from build123d import *

# Parameters (mm, degrees)
BOSS_EXTRU_1_DEPTH      = 6
ESQUISSE2_R             = 17.5
ESQUISSE2_R_2           = 1.65
ENL_V_MAT_EXTRU_1_DEPTH = 107.283818147
ENL_V_MAT_EXTRU_3_DEPTH = 107.283818147
ESQUISSE6_R             = 3.5
ENL_V_MAT_EXTRU_4_DEPTH = 4
CONG_1_R                = 20


with BuildPart() as part:
    # Esquisse1 → Boss.-Extru.1 (new body)
    with BuildSketch(Plane(origin=(0, 0, 0), x_dir=(1, 0, 0), z_dir=(0, 1, 0))):
        Polygon((-94, -35.5), (-94, -25.5), (-100, -25.5), (-100, -10.5), (-94, -10.5), (-94, 10.5), (-100, 10.5), (-100, 25.5), (-94, 25.5), (-94, 35.5), (94, 35.5), (94, 25.5), (100, 25.5), (100, 10.5), (94, 10.5), (94, -10.5), (100, -10.5), (100, -25.5), (94, -25.5), (94, -35.5), align=None)
    extrude(amount=BOSS_EXTRU_1_DEPTH)

    # Esquisse2 → Enlèv. mat.-Extru.1 (cut, through all)
    with BuildSketch(Plane(origin=(0, 0, 0), x_dir=(-1, 0, 0), z_dir=(0, -1, 0))):
        with Locations(Location((18, 11.5, 0), (0, 0, 90))):
            Circle(ESQUISSE2_R)
        with Locations(Location((71, -24.5, 0), (0, 0, 90))):
            Circle(ESQUISSE2_R_2)
        with Locations(Location((71, 25.5, 0), (0, 0, 90))):
            Circle(ESQUISSE2_R_2)
        with Locations(Location((-71, 25.5, 0), (0, 0, 270))):
            Circle(ESQUISSE2_R_2)
        with Locations(Location((-71, -24.5, 0), (0, 0, 270))):
            Circle(ESQUISSE2_R_2)
        with Locations(Location((-18, 11.5, 0), (0, 0, 270))):
            Circle(ESQUISSE2_R)
    extrude(amount=-ENL_V_MAT_EXTRU_1_DEPTH, mode=Mode.SUBTRACT)

    # Esquisse5 → Enlèv. mat.-Extru.3 (cut, through all)
    with BuildSketch(Plane.XZ):
        Polygon((-31.565369037, -0.444197772), (-18, -29), (18, -29), (31.565369037, -0.444197772), (18.743702877, 19.662334717), (-17.256297123, 19.662334717), align=None)
    extrude(amount=-ENL_V_MAT_EXTRU_3_DEPTH, mode=Mode.SUBTRACT)

    # Esquisse6 → Enlèv. mat.-Extru.4 (cut)
    with BuildSketch(Plane(origin=(0, 6, 0), x_dir=(1, 0, 0), z_dir=(0, 1, 0))):
        with Locations(Location((71, -24.5, 0), (0, 0, 270))):
            Circle(ESQUISSE6_R)
        with Locations(Location((71, 25.5, 0), (0, 0, 270))):
            Circle(ESQUISSE6_R)
        with Locations(Location((-71, 25.5, 0), (0, 0, 270))):
            Circle(ESQUISSE6_R)
        with Locations(Location((-71, -24.5, 0), (0, 0, 270))):
            Circle(ESQUISSE6_R)
    extrude(amount=-ENL_V_MAT_EXTRU_4_DEPTH, mode=Mode.SUBTRACT)

    # Congé1
    cong_1_edges = [part.edges().sort_by_distance(p)[0] for p in [
        (-17.256297123, 3, 19.662334717),
        (18.743702877, 3, 19.662334717),
    ]]
    fillet(cong_1_edges, radius=CONG_1_R)


solid = part.part
For this review, take the finished solid that the model builds, in its own axes (mm). A direction names the side the tool comes from. Round coordinates to 2 decimals unless told otherwise and drop trailing zeros. Write each loop counter-clockwise with the first axis right and the second up, starting at its lowest first coordinate (ties: lowest second). Pieces come first, ordered by that corner, then holes. Notation, with made-up numbers: M 1,-14 L 20,-14 A32 cw 20,16 Z; hole C 89.25,37.5 d5. An arc over 180 degrees is marked long. Write item = value, one per line. Start each with the question number.
(1) Clearance check with flat-ended pins moving along their axes: pin 1 Ø3 at (x, y) = (-96, 3.5) entering from -Z; pin 2 Ø2 at (x, z) = (69.5, 23.5) entering from +Y; pin 3 Ø3 at (x, z) = (-71, -25.5) entering from +Y; pin 4 Ø3 at (y, z) = (2.5, -28.5) entering from +X. State where each tip first meets the part, or that it passes through.
(2) The part is to be moulded in two halves that separate along X. For faces 6 (the face through (100, 3, 18)), 7 (the face through (97, 3, 25.5)), 8 (the face through (-33.924, 2.958, -18.759)), say which applies: +X half, -X half, draft (parallel to the pull), parting line (faces both ways), or undercut.
(3) For line 1 along Z through (x, y) = (71, 0.7); line 2 along X through (y, z) = (0.8, 24.5); line 3 along X through (y, z) = (4, 22), list the stretches that pass through material, from the lowest coordinate up.
(4) We need section C-C (z = -17). Give the boundary of the cut face in (x, y).
(5) We need section A-A (x = 4). Give the boundary of the cut face in (y, z), then the cut area to 3 significant figures.
(6) For faces 1 (the face through (33.687, 2.958, -19.258)), 2 (the face through (-94, 3, -30)), 3 (the face through (97, 3, -10.5)), 4 (the face through (-97, 3, 25.5)), 5 (the face through (69, 2, -25)), list the 3-axis set-ups (+Z, -Z, +X, -X, +Y, -Y) from which the entire face can be reached by the end or side of a thin tool; tool diameter is ignored.
(7) We need section D-D (z = 30.5). Give the boundary of the cut face in (x, y).
(8) We need section B-B (y = 1). Give the number of separate pieces and of enclosed holes in the cut face, then the cut area to 3 significant figures.
Results found:
q1.pin_1 = -25.5
q1.pin_2 = 2
q1.pin_3 = through
q1.pin_4 = 94
q2.face_6 = +X half
q2.face_7 = draft
q2.face_8 = undercut
q3.line_1 = -35.5 to -27.15, -23.85 to 22.85, 26.15 to 35.5
q3.line_2 = -100 to -72.65, -69.35 to 69.35, 72.65 to 100
q3.line_3 = -100 to -73.45, -68.55 to 68.55, 73.45 to 100
q4.outline = M -100,0 L -34.61,0 L -34.61,6 L -100,6 Z; M 34.61,0 L 100,0 L 100,6 L 34.61,6 Z
q5.outline = M 0,-35.5 L 6,-35.5 L 6,-29 L 0,-29 Z; M 0,19.66 L 6,19.66 L 6,35.5 L 0,35.5 Z
q5.area = 134 mm²
q6.face_1 = +Y, -Y
q6.face_2 = -Z, -X, +Y, -Y
q6.face_3 = +X, +Y, -Y
q6.face_4 = +Z, -X, +Y, -Y
q6.face_5 = +Y
q7.outline = M -94,0 L 94,0 L 94,6 L -94,6 Z
q8.separate_pieces = 1
q8.enclosed_holes = 5
q8.area = 10,800 mm²
